from build123d import *

# Parameters (mm, degrees)
F0_W     = 40
F0_H     = 10
F0_R     = 1.6
F1_DEPTH = 4
F2_R     = 1.5
F3_DEPTH = 1.5
F4_R     = 4.99999
F5_R     = 3
F6_DEPTH = 25
F7_R     = 6


# Not quite as in the source:
# - a fillet or chamfer is up to 0.001 mm smaller than in the source, because OpenCascade refuses the exact size


with BuildPart() as f1:
    # F0 (on Top) → F1 (new body)
    with BuildSketch(Plane.XY):
        Rectangle(F0_W, F0_H)
        with Locations((-15, 0)):
            Circle(F0_R, mode=Mode.SUBTRACT)
        with Locations((15, 0)):
            Circle(F0_R, mode=Mode.SUBTRACT)
    extrude(amount=F1_DEPTH)

    # F2 (on face) → F3 (cut)
    with BuildSketch(Plane(origin=(0, 0, 0), x_dir=(1, 0, 0), z_dir=(0, 0, -1))):
        with Locations((-7, 0)):
            Circle(F2_R)
        with Locations((7, 0)):
            Circle(F2_R)
    extrude(amount=-F3_DEPTH, mode=Mode.SUBTRACT)

    # F4 (radius 5 in the source; OpenCascade refuses exactly that, so slightly less here)
    f4_edges = [f1.edges().sort_by_distance(p)[0] for p in [
        (-20, -5, 2),
        (-20, 5, 2),
        (20, 5, 2),
        (20, -5, 2),
    ]]
    fillet(f4_edges, radius=F4_R)

    # F5 (on face) → F6 (cut)
    with BuildSketch(Plane.XY.offset(4)):
        with Locations((0, -5)):
            Circle(F5_R)
    extrude(amount=-F6_DEPTH, mode=Mode.SUBTRACT)

    # F7
    f7_edges = [f1.edges().sort_by_distance(p)[0] for p in [
        (3, -5, 2),
        (-3, -5, 2),
    ]]
    fillet(f7_edges, radius=F7_R)


solid = f1.part
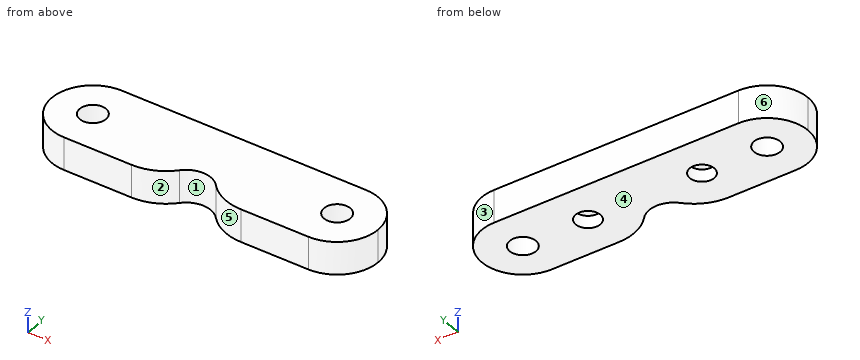
Verification items for the finished model (mm, model axes). Face numbers are marked on the shaded views. A direction names the side the tool comes from. Give positions to 0.01 mm unless a question says otherwise; leave off trailing zeros. Write each loop counter-clockwise with the first axis right and the second up, starting at its lowest first coordinate (ties: lowest second). Pieces come first, ordered by that corner, then holes. Notation, with made-up numbers: (77.25, 31.5) -> (134.25, 31.5) arc R19 cw to (134.25, 63.5) -> close; hole circle Ø2 at (1, 48). An arc over 180 degrees is marked (long way). Use CSV: the item, a comma, the result in double quotes.
(1) Material ranges on L1, parallel to Y at x = -15, z = 1.7; L2, parallel to Y at x = -7, z = 0.85; L3, parallel to X at y = 1, z = 3.85, recorded low to high.
Derived:
L1,"y = -5 to -1.6, 1.6 to 5"
L2,"y = -5 to -1.5, 1.5 to 5"
L3,"x = -19.9 to -16.25, -13.75 to 13.75, 16.25 to 19.9"
(2) Sectioned sample at B-B (y = -0.75). Record the cut outline in (x, z).
Derived:
outline,"(-19.94, 0) -> (-16.41, 0) -> (-16.41, 4) -> (-19.94, 4) -> close; (-13.59, 0) -> (-8.3, 0) -> (-8.3, 1.5) -> (-5.7, 1.5) -> (-5.7, 0) -> (5.7, 0) -> (5.7, 1.5) -> (8.3, 1.5) -> (8.3, 0) -> (13.59, 0) -> (13.59, 4) -> (-13.59, 4) -> close; (16.41, 0) -> (19.94, 0) -> (19.94, 4) -> (16.41, 4) -> close"
(3) Go/stop test with flat-tipped pins: pin 1 (1.8 mm diameter, centred on x = 7, y = 0, fed in from -Z); pin 2 (1.9 mm diameter, centred on x = -15, y = 0, fed in from +Z); pin 3 (1 mm diameter, centred on y = -2.5, z = 2.5, fed in from -X); pin 4 (1.5 mm diameter, centred on y = -2, z = 2.5, fed in from +X). Record where each tip stops, or that it passes through.
Derived:
pin 1,"stops at z = 1.5"
pin 2,"passes through"
pin 3,"stops at x = -19.58"
pin 4,"stops at x = 19.84"
(4) Sectioned sample at C-C (x = 16). Record the cut outline in (y, z), plus the area to 3 significant figures.
Derived:
outline,"(-4.9, 0) -> (-1.25, 0) -> (-1.25, 4) -> (-4.9, 4) -> close; (1.25, 0) -> (4.9, 0) -> (4.9, 4) -> (1.25, 4) -> close"
area,"29.2 mm^2"
(5) Set-up check for the marked faces 5 and 6: record each of +Z, -Z, +X, -X, +Y, -Y from which the full face is reachable in a straight line by a thin tool's end or side.
Derived:
face 5,"+Z, -Z, -Y"
face 6,"+Z, -Z, -X, +Y"
(6) Release check for a two-part mould opening along X. For the marked faces 1, 2, 3 and 4 record: +X half, -X half, draft (parallel to the pull), parting line (faces both ways), or undercut.
Derived:
face 1,"undercut"
face 2,"undercut"
face 3,"+X half"
face 4,"draft"
(7) Sectioned sample at A-A (z = 0.55). Give the number of separate pieces and of enclosed holes in the cut face, plus the area to 3 significant figures.
Derived:
separate pieces,"1"
enclosed holes,"4"
area,"331 mm^2"
